Part print with two shaded views. Sizes in mm from the minimum x, y, z corner. A direction names the side the tool comes from. Give positions to 0.01 mm unless a question says otherwise; leave off trailing zeros. Order: outer loops, then holes, each group sorted by start corner. A loop starts at its lowest first (then second) coordinate and runs counter-clockwise, first axis right, second up. Notation, with made-up numbers: (-4, 75) - (13, 75) arc R15 cw to (13, 101) - close; hole circle Ø5 at (51.25, -17.5). An arc over 180 degrees is marked (long way). Return JSON: item names as keys, results as strings. Group by question number.
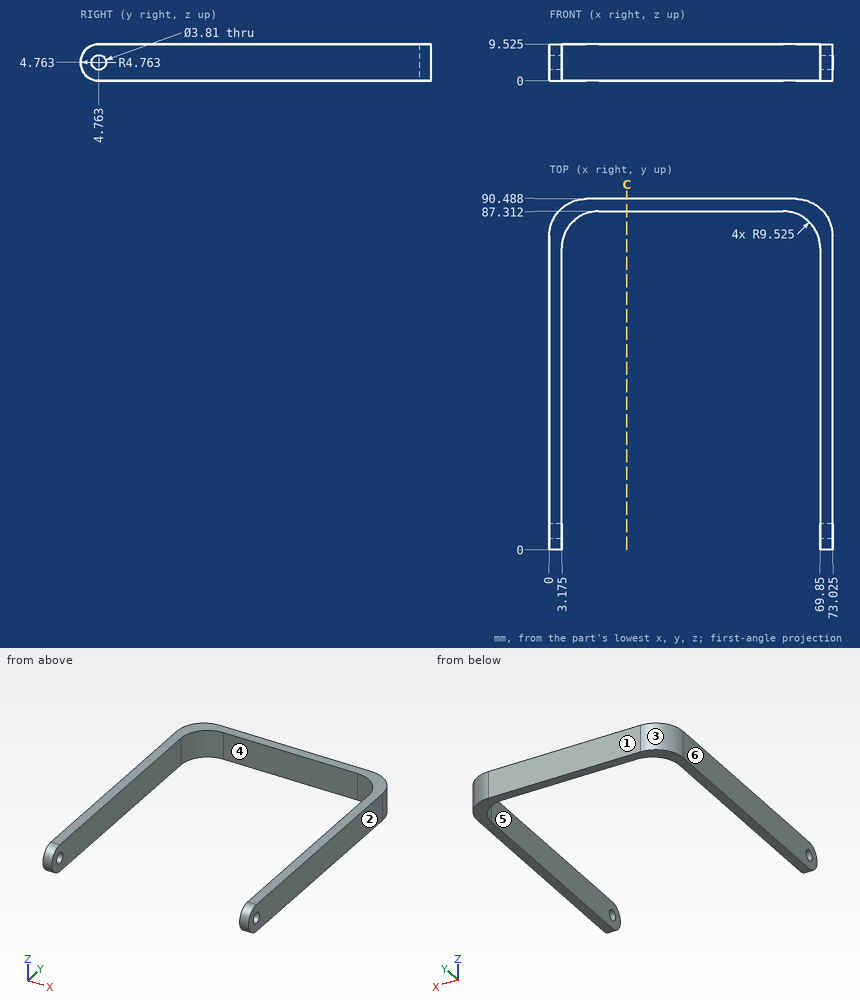
(1) Pull direction X, two halves, no side cores. Call the marked faces 1, 2, 3 and 4: released by +X, released by -X, zero draft, split by the parting line, or undercut.
(2) Slice it at C-C (x = 20). Give the cut face in (y, z) (1 decimal).
(3) 3-axis set-ups, long thin cutter, end or side, ignore diameter. For the marked faces 5 and 6: which of +Z, -Z, +X, -X, +Y, -Y reach the whole face in a straight line?
(4) Drop flat-ended pins along their axis: pin 1 Ø3 at (x, z) = (26.5, 4.5) entering from -Y; pin 2 Ø3 at (y, z) = (4.76, 4.76) entering from +X. Give the stop position or say it passes through.
(5) Drill centre lines: L1, parallel to Y at x = 27, z = 2; L2, parallel to X at y = 83.5, z = 7.5 (1 decimal); L3, parallel to X at y = 78.5, z = 7.75 (1 decimal). Where is each one in solid material? Low to high.
Result set:
{
 "1": {"face 1": "zero draft", "face 2": "released by +X", "face 3": "released by -X", "face 4": "undercut"},
 "2": {"outline": "(87.3, 0) - (90.5, 0) - (90.5, 9.5) - (87.3, 9.5) - close"},
 "3": {"face 5": "+Z, -Z, -Y", "face 6": "+Z, -Z, -X, +Y, -Y"},
 "4": {"pin 1": "stops at y = 87.31", "pin 2": "passes through"},
 "5": {"L1": "y = 87.31 to 90.49", "L2": "x = 0.3 to 5.1, 67.9 to 72.7", "L3": "x = 0 to 3.2, 69.8 to 73"}
}
